Autodesk Inventor part; units mm, degrees
ref_plane "YZ Plane" through (0, 0, 0) normal (1, 0, 0) x (0, 1, 0)
ref_plane "XZ Plane" through (0, 0, 0) normal (0, 1, 0) x (-1, 0, 0)
ref_plane "XY Plane" through (0, 0, 0) normal (0, 0, 1) x (1, 0, 0)
sketch "Skizze1" plane through (0, 0, 0) normal (0, 0, 1) x (1, 0, 0)
  line L0 (75, 38.65) -> (-75, 38.65)
  line L1 (-75, 38.65) -> (-75, -38.65)
  line L2 (-75, -38.65) -> (75, -38.65)
  line L3 (75, -38.65) -> (75, 38.65)
  line L4 (75, 38.65) -> (-75, -38.65) construction
  line L5 (-75, 38.65) -> (75, -38.65) construction
  point P0 (0, 0)
  dimension "d0" = 150
  dimension "d1" = 77.3
extrude "Extrusion1" add sketch "Skizze1" along normal blind 13.1
fillet "Rundung1" radius 2 8 edges at (0, 38.65, 13.1) (0, 38.65, 0) (0, -38.65, 13.1) (0, -38.65, 0) (75, 0, 13.1) (75, 0, 0) (-75, 0, 13.1) (-75, 0, 0)
sketch "Skizze2" plane through (-75, -38.65, 2) normal (-1, 0, 0) x (0, 0, 1)
  line L0 (0, 0) -> (0, 77.3)
  line L1 (0, 0) -> (9.1, 0)
  line L2 (9.1, 77.3) -> (9.1, 0)
  line L3 (0, 77.3) -> (9.1, 77.3)
  circle A0 centre (5.5, 15) radius 5.5
  line L4 (-2, 75.3) -> (-2, 2)
  point P0 (-2, 38.65)
  dimension "d5" = 7.5
  dimension "d6" = 15
extrude "Extrusion2" cut sketch "Skizze2" against normal blind 13.1 contours A0 L2 | A0 L2
sketch "Skizze3" plane through (-75, 38.65, 2) normal (0, 1, 0) x (1, 0, 0)
  line L0 (13.1, -11) -> (13.1, 0)
  line L1 (13.1, -7.4407) -> (35, -7.4407)
  line L2 (35, -7.4407) -> (35, -0.6533)
  line L3 (35, -0.6533) -> (13.1, -0.6533)
  line L4 (13.1, -0.6533) -> (13.1, -7.4407)
  line L5 (50, -7.4407) -> (70, -7.4407)
  line L6 (70, -7.4407) -> (70, -0.6533)
  line L7 (70, -0.6533) -> (50, -0.6533)
  line L8 (50, -0.6533) -> (50, -7.4407)
  line L9 (146.1998, -6.4555) -> (115.5466, -6.4555)
  line L10 (115.5466, -6.4555) -> (115.5466, -0.6533)
  line L11 (115.5466, -0.6533) -> (146.1998, -0.6533)
  line L12 (146.1998, -0.6533) -> (146.1998, -6.4555)
  line L13 (0, 0) -> (0, -9.1)
  point P0 (75, 2)
  dimension "d11" = 35
  dimension "d12" = 50
  dimension "d13" = 70
extrude "Extrusion3" cut sketch "Skizze3" against normal blind 13.1
sketch "Skizze4" plane through (0, 0, 13.1) normal (0, 0, 1) x (1, 0, 0)
  line L0 (-67.066, -19.0577) -> (-67.066, 14.3022) construction
  line L1 (-67.066, 14.3022) -> (-57.0354, 14.3022) construction
  line L2 (-57.0354, 14.3022) -> (-57.0354, -19.0577) construction
  line L3 (-57.0354, -19.0577) -> (-67.066, -19.0577) construction
  spline S0 degree 2 poles (-57.0666, -15.3995) (-57.0666, -16.4447) (-57.5034, -17.9111) (-57.8154, -18.5585) knots 0 0 0 1 2 2 2
  line L4 (-57.8154, -18.5585) -> (-59.4221, -18.5585)
  line L5 (-59.4221, -18.5585) -> (-59.4221, -18.4649)
  spline S1 degree 2 poles (-59.4221, -18.4649) (-58.8294, -17.8331) (-58.1742, -16.2341) (-58.1742, -15.4931) knots 0 0 0 1 2 2 2
  spline S2 degree 2 poles (-58.1742, -15.4931) (-58.1742, -14.4324) (-59.0555, -13.3482) (-59.7809, -13.3482) knots 0 0 0 1 2 2 2
  spline S3 degree 2 poles (-59.7809, -13.3482) (-60.3581, -13.3482) (-61.0757, -13.9176) (-61.2551, -14.5338) knots 0 0 0 1 2 2 2
  spline S4 degree 2 poles (-61.2551, -14.5338) (-61.3799, -14.9784) (-61.5515, -15.7193) (-61.6919, -16.2731) knots 0 0 0 1 2 2 2
  spline S5 degree 2 poles (-61.6919, -16.2731) (-61.8245, -16.7723) (-62.2223, -17.5601) (-62.5421, -17.8643) knots 0 0 0 1 2 2 2
  spline S6 degree 2 poles (-62.5421, -17.8643) (-62.8619, -18.1607) (-63.7199, -18.4883) (-64.2814, -18.4883) knots 0 0 0 1 2 2 2
  spline S7 degree 2 poles (-64.2814, -18.4883) (-65.4514, -18.4883) (-67.0348, -16.6631) (-67.0348, -15.2514) knots 0 0 0 1 2 2 2
  spline S8 degree 2 poles (-67.0348, -15.2514) (-67.0348, -14.4402) (-66.715, -13.005) (-66.4108, -12.3888) knots 0 0 0 1 2 2 2
  line L6 (-66.4108, -12.3888) -> (-64.882, -12.3888)
  line L7 (-64.882, -12.3888) -> (-64.882, -12.4824)
  spline S9 degree 2 poles (-64.882, -12.4824) (-65.3032, -12.9426) (-65.9272, -14.3778) (-65.9272, -15.1656) knots 0 0 0 1 2 2 2
  spline S10 degree 2 poles (-65.9272, -15.1656) (-65.9272, -16.0547) (-65.0926, -17.1545) (-64.414, -17.1545) knots 0 0 0 1 2 2 2
  spline S11 degree 2 poles (-64.414, -17.1545) (-63.8057, -17.1545) (-63.0803, -16.5071) (-62.9165, -15.8987) knots 0 0 0 1 2 2 2
  spline S12 degree 2 poles (-62.9165, -15.8987) (-62.8073, -15.4931) (-62.5265, -14.3154) (-62.4095, -13.9254) knots 0 0 0 1 2 2 2
  spline S13 degree 2 poles (-62.4095, -13.9254) (-62.1053, -12.9348) (-60.8807, -12.0144) (-59.9837, -12.0144) knots 0 0 0 1 2 2 2
  spline S14 degree 2 poles (-59.9837, -12.0144) (-59.4143, -12.0144) (-58.3224, -12.4746) (-57.9402, -12.888) knots 0 0 0 1 2 2 2
  spline S15 degree 2 poles (-57.9402, -12.888) (-57.519, -13.3482) (-57.0666, -14.5182) (-57.0666, -15.3995) knots 0 0 0 1 2 2 2
  spline S16 degree 2 poles (-65.7634, -3.9026) (-65.1238, -3.3566) (-63.2519, -2.7482) (-62.0507, -2.7482) knots 0 0 0 1 2 2 2
  spline S17 degree 2 poles (-62.0507, -2.7482) (-60.8807, -2.7482) (-58.9854, -3.341) (-58.3458, -3.9026) knots 0 0 0 1 2 2 2
  spline S18 degree 2 poles (-58.3458, -3.9026) (-57.675, -4.4954) (-57.0354, -6.0631) (-57.0354, -7.0069) knots 0 0 0 1 2 2 2
  spline S19 degree 2 poles (-57.0354, -7.0069) (-57.0354, -7.9819) (-57.6984, -9.5419) (-58.3458, -10.1113) knots 0 0 0 1 2 2 2
  spline S20 degree 2 poles (-58.3458, -10.1113) (-58.9854, -10.665) (-60.8651, -11.2578) (-62.0507, -11.2578) knots 0 0 0 1 2 2 2
  spline S21 degree 2 poles (-62.0507, -11.2578) (-63.2597, -11.2578) (-65.1004, -10.6572) (-65.7634, -10.1035) knots 0 0 0 1 2 2 2
  spline S22 degree 2 poles (-65.7634, -10.1035) (-66.403, -9.5419) (-67.066, -7.9741) (-67.066, -7.0069) knots 0 0 0 1 2 2 2
  spline S23 degree 2 poles (-67.066, -7.0069) (-67.066, -6.0241) (-66.3796, -4.4486) (-65.7634, -3.9026) knots 0 0 0 1 2 2 2
  spline S24 degree 2 poles (-62.0507, -4.082) (-63.0023, -4.082) (-64.4764, -4.4954) (-64.96, -4.8698) knots 0 0 0 1 2 2 2
  spline S25 degree 2 poles (-64.96, -4.8698) (-65.4592, -5.252) (-65.9584, -6.3283) (-65.9584, -6.9991) knots 0 0 0 1 2 2 2
  spline S26 degree 2 poles (-65.9584, -6.9991) (-65.9584, -7.6933) (-65.4748, -8.7385) (-64.96, -9.1363) knots 0 0 0 1 2 2 2
  spline S27 degree 2 poles (-64.96, -9.1363) (-64.4686, -9.5185) (-62.9867, -9.9241) (-62.0507, -9.9241) knots 0 0 0 1 2 2 2
  spline S28 degree 2 poles (-62.0507, -9.9241) (-60.1553, -9.9241) (-58.143, -8.3329) (-58.143, -6.9991) knots 0 0 0 1 2 2 2
  spline S29 degree 2 poles (-58.143, -6.9991) (-58.143, -5.6653) (-60.1553, -4.082) (-62.0507, -4.082) knots 0 0 0 1 2 2 2
  line L8 (-57.2382, 5.543) -> (-57.2382, 4.1078)
  line L9 (-57.2382, 4.1078) -> (-65.5372, -0.1509)
  line L10 (-65.5372, -0.1509) -> (-57.2382, -0.1509)
  line L11 (-57.2382, -0.1509) -> (-57.2382, -1.3442)
  line L12 (-57.2382, -1.3442) -> (-66.8632, -1.3442)
  line L13 (-66.8632, -1.3442) -> (-66.8632, 0.4731)
  line L14 (-66.8632, 0.4731) -> (-59.2427, 4.3496)
  line L15 (-59.2427, 4.3496) -> (-66.8632, 4.3496)
  line L16 (-66.8632, 4.3496) -> (-66.8632, 5.543)
  line L17 (-66.8632, 5.543) -> (-57.2382, 5.543)
  line L18 (-66.8632, 14.232) -> (-61.4969, 10.9795)
  line L19 (-61.4969, 10.9795) -> (-57.2382, 10.9795)
  line L20 (-57.2382, 10.9795) -> (-57.2382, 9.7003)
  line L21 (-57.2382, 9.7003) -> (-61.3643, 9.7003)
  line L22 (-61.3643, 9.7003) -> (-66.8632, 6.4478)
  line L23 (-66.8632, 6.4478) -> (-66.8632, 7.8674)
  line L24 (-66.8632, 7.8674) -> (-62.6279, 10.3477)
  line L25 (-62.6279, 10.3477) -> (-66.8632, 12.8749)
  line L26 (-66.8632, 12.8749) -> (-66.8632, 14.232)
  point P0 (0, 0)
extrude "Extrusion4" cut sketch "Skizze4" against normal blind 1
properties part number "00_Sony_MDL_Projector"
The listing builds one solid part. Answer for the finished solid, in the listing's coordinates (mm). A direction names the side the tool comes from. Coordinates: 2 decimals unless noted, no trailing zeros. Answer as a JSON object with one key per item and string values. Group by question number.
Item 1: Which of the six approach directions +Z, -Z, +X, -X, +Y, -Y give full straight-line access (tool end or side, diameter ignored) to faces 1 (the face through (-63.106, 2.384, 12.607)), 2 (the face through (-15, 32, 9.441)), 3 (the face through (-1, 1, 13.1))?
Item 2: Consider L1, parallel to Y at x = -71.5, z = 7.5; L2, parallel to Y at x = -12, z = 3.25; L3, parallel to X at y = -24, z = 6.75. Determine where each line is inside the solid, lowest interval first.
Item 3: Each of these flat-tipped pins is pushed along its axis until it touches: P1, Ø6.5, axis at y = -23.65, z = 7.5, coming from the -X side; P2, Ø1.5, axis at x = 10, y = 8, coming from the -Z side; P3, Ø0.5, axis at x = -60.5, z = 12.5, coming from the +Y side; P4, Ø0.8, axis at x = -59.5, z = 12.5, coming from the +Y side. Where does it stop, or does it pass through?
Item 4: Determine the mould class of faces 4 (the face through (-64.075, 8.097, 12.607)), 5 (the face through (-51, 32, 9.441)), 6 (the face through (-61, -4, 12.1)) for opening direction Z: +Z half, -Z half, draft (parallel to the pull), parting line (faces both ways), or undercut.
Solved:
{
 "1": {"face 1": "+Z", "face 2": "+Y", "face 3": "+Z, +X, -X, +Y, -Y"},
 "2": {"L1": "y = -38.65 to -29.15, -18.15 to 38.65", "L2": "y = -38.65 to 25.55", "L3": "x = -61.9 to 75"},
 "3": {"P1": "stops at x = -61.9", "P2": "stops at z = 0", "P3": "stops at y = 38.29", "P4": "stops at y = 38.38"},
 "4": {"face 4": "draft", "face 5": "undercut", "face 6": "+Z half"}
}
